Geometry check sheet. Reference: the model listing, model coordinates, mm. A direction names the side the tool comes from. Coordinates: 2 decimals unless noted, no trailing zeros. Write each loop counter-clockwise with the first axis right and the second up, starting at its lowest first coordinate (ties: lowest second). Pieces come first, ordered by that corner, then holes. Notation, with made-up numbers: M 68,28.5 L 113,28.5 A23 ccw 113,62.5 Z; hole C 66.5,-22.75 d11. An arc over 180 degrees is marked long. Write each question's results on one line, items separated by ' | '.
```python
from build123d import *

# Parameters (mm, degrees)
F0_W     = 1800
F0_H     = 900
F1_DEPTH = 5
F2_W     = 10
F2_H     = 900
F3_DEPTH = 1800
F5_DEPTH = 1800.001
F7_D     = 12


with BuildPart() as f1:
    # F0 (on Front) → F1 (new body, symmetric)
    with BuildSketch(Plane.XZ):
        Rectangle(F0_W, F0_H)
    extrude(amount=F1_DEPTH, both=True)

    # F2 (on face) → F3 (join)
    with BuildSketch(Plane.XZ.offset(5)):
        with Locations((-895, 0)):
            Rectangle(F2_W, F2_H)
        with Locations((895, 0)):
            Rectangle(F2_W, F2_H)
    extrude(amount=F3_DEPTH)

    # F4 (on face) → F5 (cut, through all)
    with BuildSketch(Plane.YZ.offset(900)):
        Polygon((-905, -450), (-1805, 450), (-1805, -450), align=None)
    extrude(amount=-F5_DEPTH, mode=Mode.SUBTRACT)

    # F7 (through all)
    with Locations(Plane(origin=(-900, 0, 0), x_dir=(0, -1, 0), z_dir=(-1, 0, 0))):
        with Locations((270, 400), (55, -213.412585)):
            Hole(F7_D / 2)


solid = f1.part
```
Q1. Sectioned sample at D-D on x = 253.5. Record the cut outline in (y, z), and give its area (3 significant figures).
Geometry check:
outline: M -5,-450 L 5,-450 L 5,450 L -5,450 Z | area: 9,000 mm2
Q2. Access from +Z, -Z, +X, -X, +Y, -Y to the whole of each face (thin tool, end or side, straight path). Record for faces 4 (the flat face through (-13, 5, 6)), 5 (the flat face through (-890, -692, -6)).
Geometry check:
face 4: +Z, -Z, +X, -X, +Y | face 5: +Z, -Z, -Y
Q3. Sectioned sample at C-C on y = -1244.5. Record the cut outline in (x, z).
Geometry check:
outline: M -900,-110.5 L -890,-110.5 L -890,450 L -900,450 Z; M 890,-110.5 L 900,-110.5 L 900,450 L 890,450 Z
Q4. Mould release check, pull along X, two halves, no side actions. Record for faces 1 (the flat face through (895, -1349, -6)), 2 (the flat face through (890, -692, -6)), 3 (the flat face through (900, -712, -6)): pulls with the +X half, pulls with the -X half, needs draft (parallel to the pull), parting line crosses it, or undercut.
Geometry check:
face 1: needs draft | face 2: undercut | face 3: pulls with the +X half
Q5. Sectioned sample at B-B on z = -179. Record the cut outline in (x, y).
Geometry check:
outline: M -900,-1176 L -890,-1176 L -890,-5 L 890,-5 L 890,-1176 L 900,-1176 L 900,5 L -900,5 Z
Q6. Sectioned sample at A-A on y = -390.5. Record the cut outline in (x, z), and give its area (3 significant figures).
Geometry check:
outline: M -900,-450 L -890,-450 L -890,450 L -900,450 Z; M 890,-450 L 900,-450 L 900,450 L 890,450 Z | area: 18,000 mm2
Q7. Scan lines: probe 1 along X at (y, z) = (-1059.5, 204); probe 2 along Z at (x, y) = (-896, -270); probe 3 along Y at (x, z) = (-326, 20.5). Record each from-to range of solid material in increasing order.
Geometry check:
probe 1: x = -900 to -890, 890 to 900 | probe 2: z = -450 to 394, 406 to 450 | probe 3: y = -5 to 5
Q8. Depth check by flat-ended pin: P1, Ø11, axis at y = -270, z = 400, coming from the -X side; P2, Ø3, axis at x = 691, z = -318, coming from the -Y side. Enter the tip coordinate at first touch or a pass-through.
Geometry check:
P1: passes through | P2: stops at y = -5
